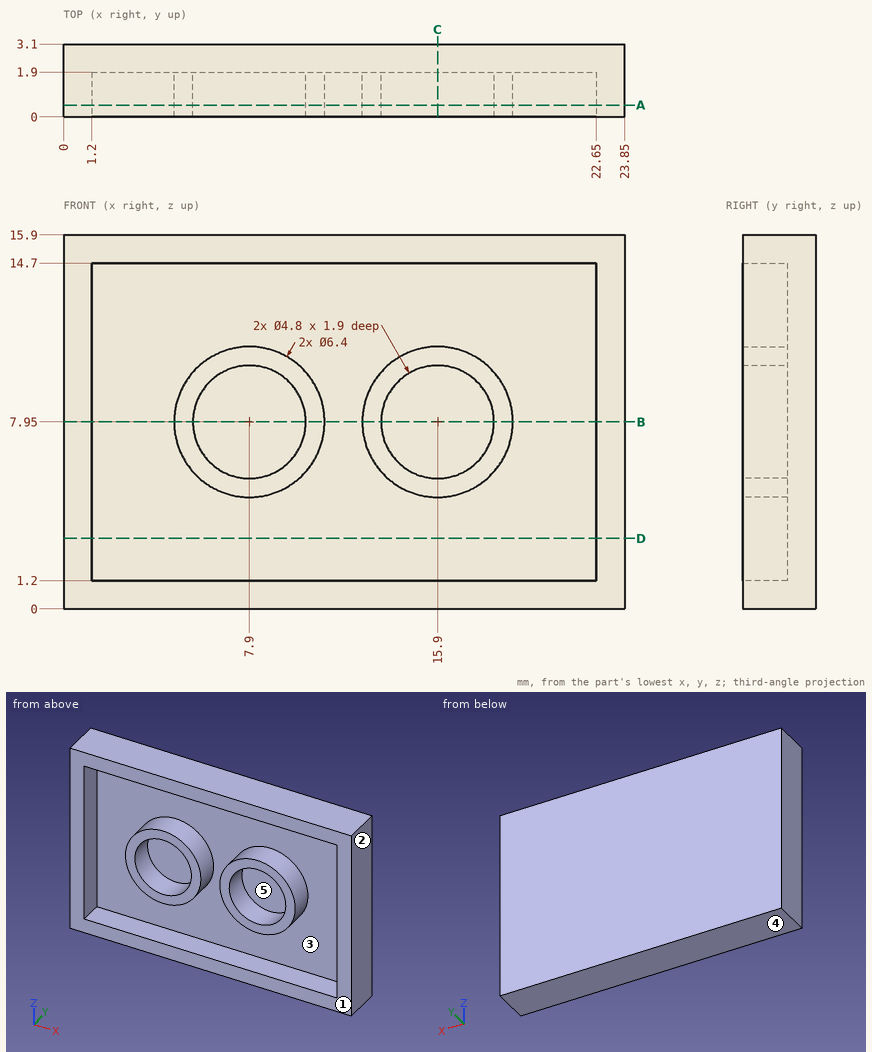
Job drawing, mm, ordinate dimensions from the low corner. One solid piece. A direction names the side the tool comes from. Give positions to 0.01 mm unless a question says otherwise; leave off trailing zeros. Write each loop counter-clockwise with the first axis right and the second up, starting at its lowest first coordinate (ties: lowest second). Pieces come first, ordered by that corner, then holes. Notation, with made-up numbers: (22, 72) - (35, 72) arc R29 cw to (35, 103) - close; hole circle Ø3 at (-2, -9). An arc over 180 degrees is marked (long way). Use one line per item in the form item = value. Start each with the question number.
1. Band-saw the part on C-C on x = 15.9. Write the cut outline in (y, z).
2. Band-saw the part on D-D on z = 3. Write the cut outline in (x, y).
3. Band-saw the part on A-A on y = 0.5. Write the cut outline in (x, z), plus the area to 3 significant figures.
4. Drop a flat-ended pin along its axis: pin 1 Ø4.5 at (x, z) = (7.9, 7.95) entering from -Y. Give the stop position or say it passes through.
5. 3-axis set-ups, long thin cutter, end or side, ignore diameter. For the marked faces 4 and 5: which of +Z, -Z, +X, -X, +Y, -Y reach the whole face in a straight line?
6. Two-plate mould, pull along X, no slides. Class the marked faces 1, 2 and 3: released by +X, released by -X, zero draft, split by the parting line, or undercut.
7. Band-saw the part on B-B on z = 7.95. Write the cut outline in (x, y).
8. Probe line 1 (X direction, y = 1.4, z = 7.95); line 2 (Z direction, x = 10, y = 1.8). List the from-to ranges inside material, lowest first. Write a range as [from, to].
Conclusion:
q1.outline = (0, 0) - (3.1, 0) - (3.1, 15.9) - (0, 15.9) - (0, 14.7) - (1.9, 14.7) - (1.9, 11.15) - (0, 11.15) - (0, 10.35) - (1.9, 10.35) - (1.9, 5.55) - (0, 5.55) - (0, 4.75) - (1.9, 4.75) - (1.9, 1.2) - (0, 1.2) - close
q2.outline = (0, 0) - (1.2, 0) - (1.2, 1.9) - (22.65, 1.9) - (22.65, 0) - (23.85, 0) - (23.85, 3.1) - (0, 3.1) - close
q3.outline = (0, 0) - (23.85, 0) - (23.85, 15.9) - (0, 15.9) - close; circle Ø6.4 at (7.9, 7.95); circle Ø6.4 at (15.9, 7.95); hole (1.2, 1.2) - (22.65, 1.2) - (22.65, 14.7) - (1.2, 14.7) - close; hole circle Ø4.8 at (7.9, 7.95); hole circle Ø4.8 at (15.9, 7.95)
q3.area = 118 mm²
q4.pin_1 = 1.9
q5.face_4 = -Z, +X, -X, +Y, -Y
q5.face_5 = -Y
q6.face_1 = zero draft
q6.face_2 = released by +X
q6.face_3 = undercut
q7.outline = (0, 0) - (1.2, 0) - (1.2, 1.9) - (4.7, 1.9) - (4.7, 0) - (5.5, 0) - (5.5, 1.9) - (10.3, 1.9) - (10.3, 0) - (11.1, 0) - (11.1, 1.9) - (12.7, 1.9) - (12.7, 0) - (13.5, 0) - (13.5, 1.9) - (18.3, 1.9) - (18.3, 0) - (19.1, 0) - (19.1, 1.9) - (22.65, 1.9) - (22.65, 0) - (23.85, 0) - (23.85, 3.1) - (0, 3.1) - close
q8.line_1 = [0, 1.2], [4.7, 5.5], [10.3, 11.1], [12.7, 13.5], [18.3, 19.1], [22.65, 23.85]
q8.line_2 = [0, 1.2], [5.54, 6.79], [9.11, 10.36], [14.7, 15.9]
